from build123d import *

# Parameters (mm, degrees)
SKETCH1_W               = 60
SKETCH1_H               = 35
BOSS_EXTRUDE1_DEPTH     = 13
CUT_EXTRUDE1_DEPTH      = 64.837684937
CUT_EXTRUDE1_DEPTH_BACK = 64.837684937
SKETCH3_R               = 1.75
SKETCH4_W               = 60
SKETCH4_H               = 3
CUT_EXTRUDE2_DEPTH      = 1
SKETCH5_R               = 1.75
CUT_EXTRUDE3_DEPTH      = 38.084363362
CHAMFER1_SIZE           = 5
SKETCH6_R               = 3.75
CUT_EXTRUDE4_DEPTH      = 7
CHAMFER2_SIZE           = 0.5


with BuildPart() as part:
    # Sketch1 → Boss-Extrude1 (new body)
    with BuildSketch(Plane.XY):
        Rectangle(SKETCH1_W, SKETCH1_H)
    extrude(amount=BOSS_EXTRUDE1_DEPTH)

    # Sketch2 → Cut-Revolve1 (revolve, cut)
    with BuildSketch(Plane.XY.offset(13)):
        with BuildLine():
            Line((-25, 0), (-25, 8.218127455))
            ThreePointArc((-25, 8.218127455), (-24.486963528, 9.469250598), (-23.243251097, 10))
            ThreePointArc((-23.243251097, 10), (-15.040879193, 9.611248064), (-6.94833646, 8.218127455))
            ThreePointArc((-6.94833646, 8.218127455), (0, 7.408356031), (6.94833646, 8.218127455))
            ThreePointArc((6.94833646, 8.218127455), (15.040879193, 9.611248064), (23.243251097, 10))
            ThreePointArc((23.243251097, 10), (24.486963528, 9.469250598), (25, 8.218127455))
            Line((25, 8.218127455), (25, 0))
            Line((25, 0), (-25, 0))
        make_face()
    revolve(axis=Axis((25, 0, 13), (-1, 0, 0)), mode=Mode.SUBTRACT)

    # Sketch3 → Cut-Extrude1 (cut, two sides: drawn at the far end of the back side and taken through both)
    with BuildSketch(Plane(origin=(30, 0, 0), x_dir=(0, 0, -1), z_dir=(1, 0, 0)).offset(-CUT_EXTRUDE1_DEPTH_BACK)):
        with Locations((-13, 0)):
            Circle(SKETCH3_R)
    extrude(amount=CUT_EXTRUDE1_DEPTH + CUT_EXTRUDE1_DEPTH_BACK, mode=Mode.SUBTRACT)

    # Sketch4 → Cut-Extrude2 (cut)
    with BuildSketch(Plane.XY.offset(13)):
        with Locations((0, 16)):
            Rectangle(SKETCH4_W, SKETCH4_H)
        with Locations((0, -16)):
            Rectangle(SKETCH4_W, SKETCH4_H)
    extrude(amount=-CUT_EXTRUDE2_DEPTH, mode=Mode.SUBTRACT)

    # Sketch5 → Cut-Extrude3 (cut, through all)
    with BuildSketch(Plane.XY.offset(13)):
        with Locations((0, 11.25)):
            Circle(SKETCH5_R)
        with Locations((0, -11.25)):
            Circle(SKETCH5_R)
    extrude(amount=-CUT_EXTRUDE3_DEPTH, mode=Mode.SUBTRACT)

    # Chamfer1
    chamfer1_edges = [part.edges().sort_by_distance(p)[0] for p in [
        (-30, 0, 0),
        (30, 0, 0),
    ]]
    chamfer(chamfer1_edges, length=CHAMFER1_SIZE)

    # Sketch6 → Cut-Extrude4 (cut)
    with BuildSketch(Plane(origin=(0, 0, 0), x_dir=(-1, 0, 0), z_dir=(0, 0, -1))):
        with Locations((0, 11.25)):
            Circle(SKETCH6_R)
        with Locations((0, -11.25)):
            Circle(SKETCH6_R)
    extrude(amount=-CUT_EXTRUDE4_DEPTH, mode=Mode.SUBTRACT)

    # Chamfer2
    chamfer2_edges = [part.edges().sort_by_distance(p)[0] for p in [
        (3.75, -11.25, 0),
        (3.75, -11.25, 7),
        (-1.75, -11.25, 7),
        (3.75, 11.25, 0),
        (3.75, 11.25, 7),
        (-1.75, 11.25, 7),
    ]]
    chamfer(chamfer2_edges, length=CHAMFER2_SIZE)


solid = part.part
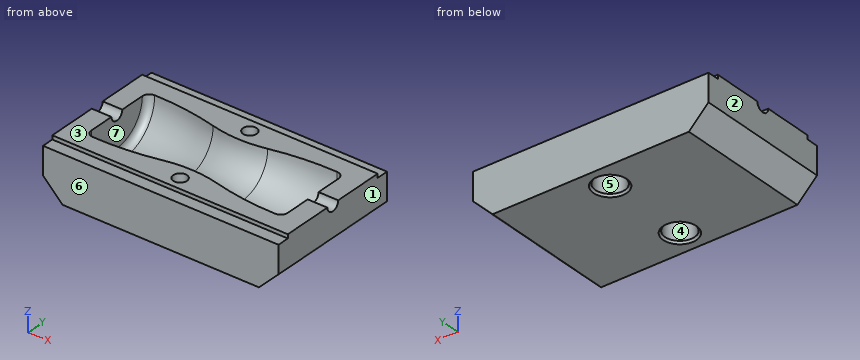
Read the model definition and answer for the solid it produces. Units are mm, in the model's axes. Face numbers are marked on the shaded views. A direction names the side the tool comes from. Round coordinates to 2 decimals unless told otherwise and drop trailing zeros. Order: outer loops, then holes, each group sorted by start corner. A loop starts at its lowest first (then second) coordinate and runs counter-clockwise, first axis right, second up.
1) Flat-ended cylindrical pins translate along their axes: pin 1 (2 mm diameter, centred on x = 0, y = 11.5, fed in from -Z); pin 2 (0.5 mm diameter, centred on x = 7, z = 12.5, fed in from -Y); pin 3 (3.5 mm diameter, centred on x = 12.5, y = -16.5, fed in from +Z); pin 4 (5 mm diameter, centred on x = -1.5, y = -10.5, fed in from -Z). Find the tip coordinate at first contact, or state that the pin passes through.
2) The mould has two halves that part along X. Classify the marked faces 1, 2, 3 and 4: released by +X, released by -X, zero draft, split by the parting line, or undercut.
3) Straight lines are drawn through the part: L1, parallel to Y at x = 0, z = 2.2; L2, parallel to Y at x = 0, z = 11.55; L3, parallel to X at y = -1.5, z = 12. For each, find the intervals that lie inside material, in ascending order.
4) The part is cut by section A-A on y = -11.25. Write down the section's boundary in (x, z), plus the area to 3 significant figures.
5) The part is cut by section B-B on x = 0. Give the number of separate pieces and of enclosed holes in the cut face, plus the area to 3 significant figures.
6) For the marked faces 5, 6 and 7, determine the directions among +Z, -Z, +X, -X, +Y, -Y from which every point of the face is accessible in a straight line to the end or side of a thin tool.
Resolved:
1. pin 1: passes through
1. pin 2: stops at y = -14.5
1. pin 3: stops at z = 12
1. pin 4: stops at z = 0.07
2. face 1: released by +X
2. face 2: released by -X
2. face 3: zero draft
2. face 4: undercut
3. L1: y = -17.5 to -15, -7.5 to 7.5, 15 to 17.5
3. L2: y = -17.5 to -13, -9.5 to -7.27, 7.27 to 9.5, 13 to 17.5
3. L3: x = -30 to -25, 25 to 30
4. outline: (-30, 5) - (-25, 0) - (-4.25, 0) - (-3.75, 0.5) - (-3.75, 6.5) - (-3.25, 7) - (-2.25, 7) - (-1.75, 7.5) - (-1.75, 13) - (-30, 13) - close; (1.75, 7.5) - (2.25, 7) - (3.25, 7) - (3.75, 6.5) - (3.75, 0.5) - (4.25, 0) - (25, 0) - (30, 5) - (30, 13) - (1.75, 13) - close
4. area: 681 mm2
5. separate pieces: 3
5. enclosed holes: 0
5. area: 215 mm2
6. face 5: -Z
6. face 6: +Z, -Z, +X, -X, -Y
6. face 7: +Z
